Check sheet for the drawn part. Datum: minimum x, y, z corner. Units: mm. A direction names the side the tool comes from. Round coordinates to 2 decimals unless told otherwise and drop trailing zeros. Write each loop counter-clockwise with the first axis right and the second up, starting at its lowest first coordinate (ties: lowest second). Pieces come first, ordered by that corner, then holes. Notation, with made-up numbers: (12.25, 88.25) -> (54.25, 88.25) arc R23 ccw to (54.25, 99.25) -> close; hole circle Ø9 at (88, 28). An arc over 180 degrees is marked (long way). Use a Markdown table: item, result.
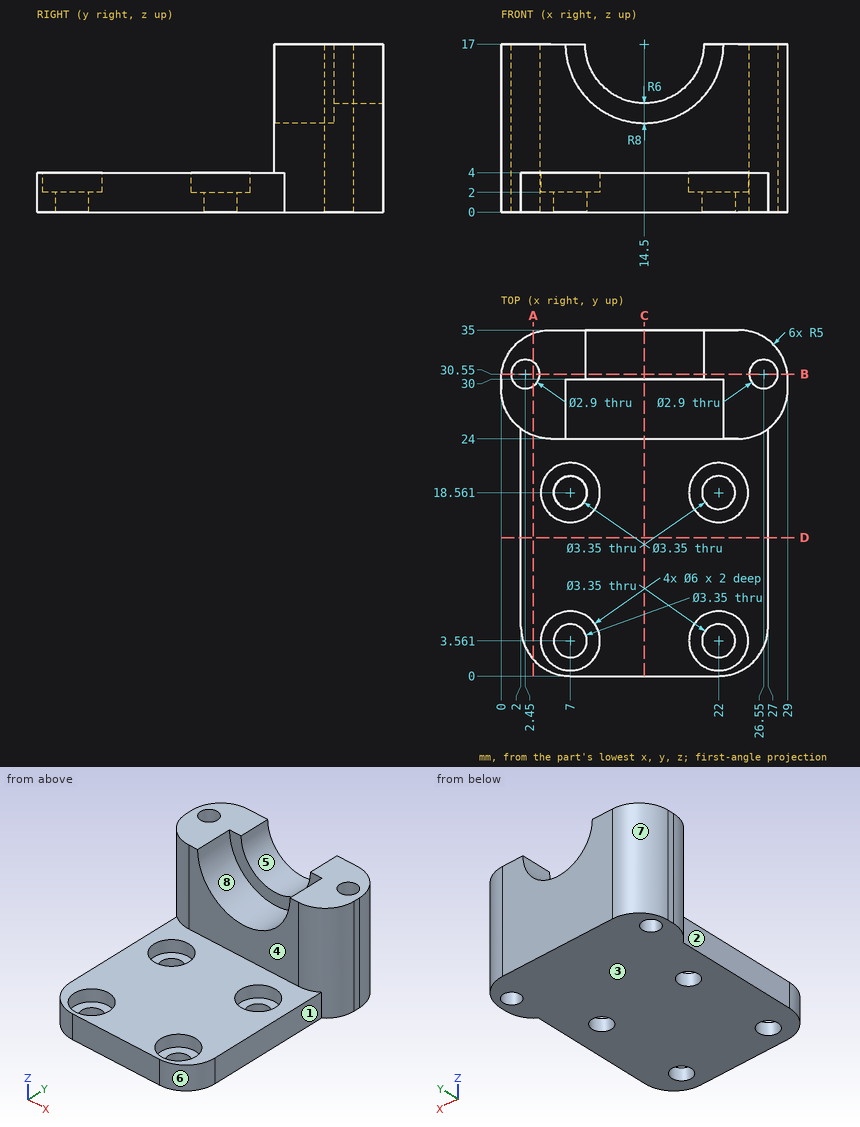
(1) Access from +Z, -Z, +X, -X, +Y, -Y to the whole of each face (thin tool, end or side, straight path). Record for the marked faces 1, 2, 3 and 4.
A:
| item | result |
|---|---|
| face 1 | +Z, -Z, +X, -Y |
| face 2 | +Z, -Z, -X, -Y |
| face 3 | -Z, +X, -X, +Y, -Y |
| face 4 | +Z, +X, -X, -Y |
(2) Section check D-D on y = 14. Record the cut outline in (x, z).
A:
| item | result |
|---|---|
| outline | (2, 0) -> (27, 0) -> (27, 4) -> (2, 4) -> close |
(3) Section check B-B on y = 30.55. Record the cut outline in (x, z).
A:
| item | result |
|---|---|
| outline | (0.03, 0) -> (1, 0) -> (1, 17) -> (0.03, 17) -> close; (3.9, 0) -> (25.1, 0) -> (25.1, 17) -> (20.5, 17) arc R6 cw to (8.5, 17) -> (3.9, 17) -> close; (28, 0) -> (28.97, 0) -> (28.97, 17) -> (28, 17) -> close |
(4) Release check for a two-part mould opening along X. For the marked faces 5, 6, 7 and 8 record: +X half, -X half, draft (parallel to the pull), parting line (faces both ways), or undercut.
A:
| item | result |
|---|---|
| face 5 | undercut |
| face 6 | +X half |
| face 7 | -X half |
| face 8 | undercut |
(5) Section check A-A on x = 3.25. Record the cut outline in (y, z).
A:
| item | result |
|---|---|
| outline | (1.69, 0) -> (29.34, 0) -> (29.34, 17) -> (24.32, 17) -> (24.32, 4) -> (1.69, 4) -> close; (31.76, 0) -> (34.68, 0) -> (34.68, 17) -> (31.76, 17) -> close |
(6) Section check C-C on x = 14.5. Record the cut outline in (y, z), plus the area to 3 significant figures.
A:
| item | result |
|---|---|
| outline | (0, 0) -> (35, 0) -> (35, 11) -> (30, 11) -> (30, 9) -> (24, 9) -> (24, 4) -> (0, 4) -> close |
| area | 205 mm2 |
(7) Thickness scan on line 1 (Y direction, x = 22, z = 2.6); line 2 (Y direction, x = 22, z = 0.85) (1 decimal); line 3 (X direction, y = 31.5, z = 1.5) (1 decimal). Record the ranges inside material, lowest first.
A:
| item | result |
|---|---|
| line 1 | y = 0 to 0.56, 6.56 to 15.56, 21.56 to 35 |
| line 2 | y = 0 to 1.9, 5.2 to 16.9, 20.2 to 35 |
| line 3 | x = 0.2 to 1.4, 3.5 to 25.5, 27.6 to 28.8 |
(8) Gauge pin test, flat ends, axial feed: pin 1 Ø1.5 at (x, y) = (16, 10.5) entering from +Z; pin 2 Ø1.8 at (x, y) = (21.5, 4) entering from +Z; pin 3 Ø3 at (x, y) = (7, 4.5) entering from +Z; pin 4 Ø6.5 at (x, z) = (12, 13.5) entering from -Y. Record the tip position at first contact, or that the pin passes through.
A:
| item | result |
|---|---|
| pin 1 | stops at z = 4 |
| pin 2 | passes through |
| pin 3 | stops at z = 2 |
| pin 4 | stops at y = 30 |
